Geometry: see drawing. Coordinates: mm, zero at the bounding-box minimum. A direction names the side the tool comes from. Coordinates: 2 decimals unless noted, no trailing zeros. Write each loop counter-clockwise with the first axis right and the second up, starting at its lowest first coordinate (ties: lowest second). Pieces come first, ordered by that corner, then holes.
1) Set-up query: the marked faces 3 and 4. Return all of +Z, -Z, +X, -X, +Y, -Y with unobstructed straight access to the full face (end or side cutting, diameter ignored); none if empty.
2) Draft query along X for the marked faces 1 and 2. Return one class per face: pulls with the +X half, pulls with the -X half, needs draft (parallel to the pull), parting line crosses it, or undercut.
3) Section query A-A (y = 10). Output: boundary loops of the cut face in (x, z), then the cut area to 3 significant figures.
4) Line query: L1, parallel to Y at x = 13.25, z = 1.55; L2, parallel to X at y = 10.25, z = 2.05; L3, parallel to Z at x = 8, y = 17.25. Output: solid intervals per line, ascending.
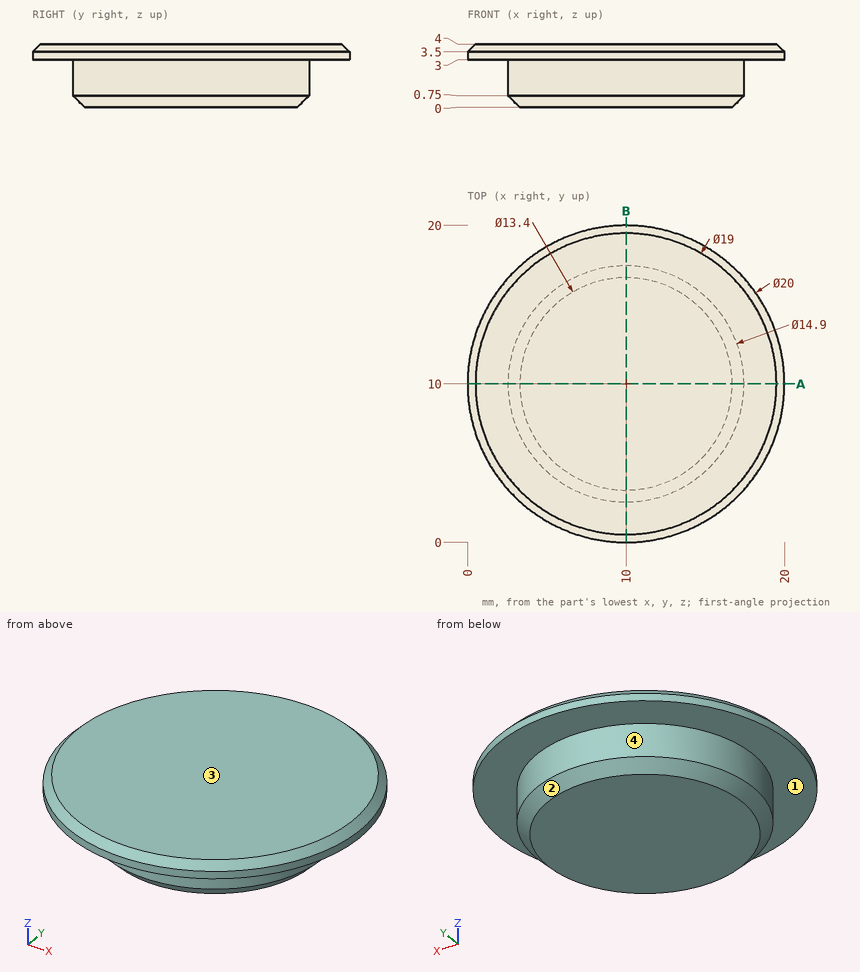
Answer:
1. face 3: +Z, +X, -X, +Y, -Y
1. face 4: -Z
2. face 1: needs draft
2. face 2: parting line crosses it
3. outline: (0, 3) - (2.55, 3) - (2.55, 0.75) - (3.3, 0) - (16.7, 0) - (17.45, 0.75) - (17.45, 3) - (20, 3) - (20, 3.5) - (19.5, 4) - (0.5, 4) - (0, 3.5) - close
3. area: 63.9 mm2
4. L1: y = 3.3 to 16.7
4. L2: x = 2.55 to 17.45
4. L3: z = 3 to 4
